Part print with two shaded views. Sizes in mm from the minimum x, y, z corner. A direction names the side the tool comes from. Give positions to 0.01 mm unless a question says otherwise; leave off trailing zeros. Write each loop counter-clockwise with the first axis right and the second up, starting at its lowest first coordinate (ties: lowest second). Pieces come first, ordered by that corner, then holes. Notation, with made-up numbers: (33, -21) - (88, -21) arc R19 cw to (88, 3) - close; hole circle Ø4 at (-23, 13.5). An arc over 180 degrees is marked (long way). One line per item, written item: value. Start each with the question number.
(1) Cut at D-D, the plane x = 23.5. List the corners of the cut face in (y, z).
(2) 3-axis set-ups, long thin cutter, end or side, ignore diameter. For the marked faces 1, 2, 3, 4 and 5: which of +Z, -Z, +X, -X, +Y, -Y reach the whole face in a straight line?
(3) Drop flat-ended pins along their axis: P1, Ø1.9, axis at x = 24.5, z = 5.5, coming from the +Y side; P2, Ø2, axis at x = 1.88, z = 3.805, coming from the -Y side; P3, Ø4, axis at x = 12, z = 1.5, coming from the +Y side. Give the stop position or say it passes through.
(4) Cut at B-B, the plane y = 12. List the corners of the cut face in (x, z) (1 decimal), and give its area (3 significant figures).
(5) Cut at A-A, the plane x = 1.88. List the corners of the cut face in (y, z) (1 decimal).
(6) Cut at C-C, the plane z = 5.75. List the corners of the cut face in (x, y).
(7) Probe L1, parallel to Z at x = 1.88, y = 11.75 (1 decimal); L2, parallel to X at y = 4.5, z = 4; L3, parallel to Y at x = 5.5, z = 1.75. List the from-to ranges inside material, lowest first.
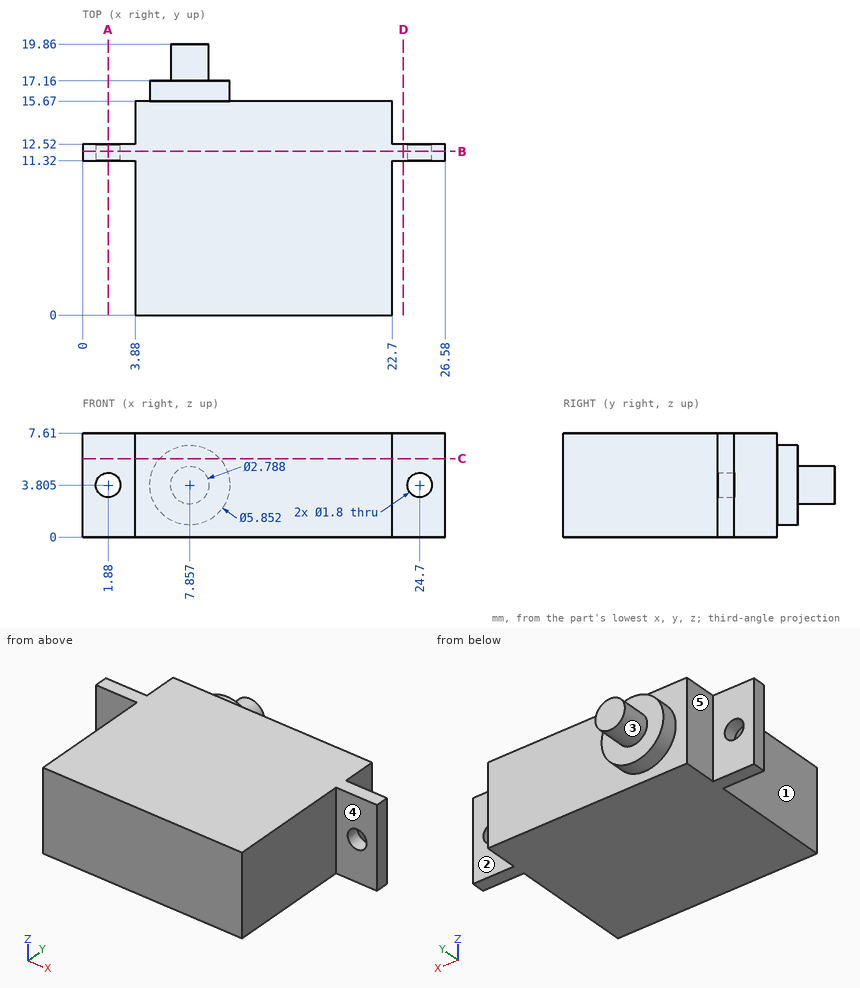
Answers follow:
1. outline: (11.32, 0) - (12.52, 0) - (12.52, 7.61) - (11.32, 7.61) - close
2. face 1: +Z, -Z, -X, -Y
2. face 2: +Z, -Z, +X, +Y
2. face 3: +Y
2. face 4: +Z, -Z, +X, -Y
2. face 5: +Z, -Z, -X, +Y
3. P1: stops at y = 12.52
3. P2: stops at y = 11.32
3. P3: stops at y = 17.16
4. outline: (0, 0) - (26.6, 0) - (26.6, 7.6) - (0, 7.6) - close; hole circle Ø1.8 at (1.9, 3.8); hole circle Ø1.8 at (24.7, 3.8)
4. area: 197 mm²
5. outline: (11.3, 0) - (12.5, 0) - (12.5, 2.9) - (11.3, 2.9) - close; (11.3, 4.7) - (12.5, 4.7) - (12.5, 7.6) - (11.3, 7.6) - close
6. outline: (0, 11.32) - (3.88, 11.32) - (3.88, 0) - (22.7, 0) - (22.7, 11.32) - (26.58, 11.32) - (26.58, 12.52) - (22.7, 12.52) - (22.7, 15.67) - (10.04, 15.67) - (10.04, 17.16) - (5.67, 17.16) - (5.67, 15.67) - (3.88, 15.67) - (3.88, 12.52) - (0, 12.52) - close
7. L1: z = 0 to 2.9, 4.7 to 7.6
7. L2: x = 3.88 to 22.7
7. L3: y = 0 to 15.67
